Read the model definition and answer for the solid it produces. Units are mm, in the model's axes. A direction names the side the tool comes from. Coordinates: 2 decimals unless noted, no trailing zeros. Order: outer loops, then holes, each group sorted by start corner. A loop starts at its lowest first (then second) coordinate and runs counter-clockwise, first axis right, second up. Notation, with made-up numbers: M -39,-39.75 L -4,-39.75 A8 cw -4,-28.75 Z; hole C 63.25,75 d9. An arc over 180 degrees is marked long. Use a Markdown table: item, result. Add a question column.
1) Find the intervals of material crossed by probe 1 along X at (y, z) = (2, -15); probe 2 along X at (y, z) = (-17, 2.5); probe 3 along X at (y, z) = (1, -6), in increasing order. Write a range as [from, to].
2) Each of these flat-tipped pins is pushed along its axis until it touches: pin 1 Ø2 at (x, z) = (14, -32) entering from -Y; pin 2 Ø9 at (x, z) = (0, -6) entering from +Y; pin 3 Ø4.5 at (x, z) = (-19, -22.5) entering from -Y; pin 4 Ø3 at (y, z) = (-1, -11) entering from -X. Where does it stop, or does it pass through?
3) For faces 5 (the face through (0, 0, -19)), 6 (the face through (24, 11, -35)), 7 (the face through (31.5, 26, 7)), determine the directions among +Z, -Z, +X, -X, +Y, -Y from which every point of the face is accessible in a straight line to the end or side of a thin tool.
4) The mould has two halves that part along Z. Classify faces 1 (the face through (-0.05, -27.25, 3.97)), 2 (the face through (-1.05, 1.6, -3.46)), 3 (the face through (-8, -13, 6)), 4 (the face through (26, 26, 5.5)): released by +Z, released by -Z, zero draft, split by the parting line, or undercut.
5) Find section A-A on y = -22. Write down the section's boundary in (x, z), plus the area to 3 significant figures.
6) Find section D-D on y = 33. Write down the section's boundary in (x, z).
7) Find section C-C on z = -22.5. Write down the section's boundary in (x, y).
8) Find section B-B on x = -19. Write down the section's boundary in (y, z), plus the area to 3 significant figures.
from build123d import *

# Parameters (mm, degrees)
SKETCH1_R           = 2.75
SKETCH1_R_2         = 2.25
BOSS_EXTRUDE1_DEPTH = 4
SKETCH3_W           = 10
SKETCH3_H           = 10
BOSS_EXTRUDE3_DEPTH = 15
SKETCH4_R           = 2.5
CUT_EXTRUDE1_DEPTH  = 58.280013966
CHAMFER1_SIZE       = 0.75
SKETCH5_W           = 4
SKETCH5_H           = 34
BOSS_EXTRUDE4_DEPTH = 68
SKETCH7_R           = 2.75
CUT_EXTRUDE2_DEPTH  = 62.806148561
CHAMFER2_SIZE       = 0.5
SKETCH8_W           = 15
SKETCH8_H           = 10
BOSS_EXTRUDE5_DEPTH = 110
CUT_EXTRUDE3_DEPTH  = 99.346326825
SKETCH10_W          = 10
SKETCH10_H          = 3
CUT_EXTRUDE4_DEPTH  = 122.885191882


with BuildPart() as part:
    # Sketch1 → Boss-Extrude1 (new body)
    with BuildSketch(Plane(origin=(0, 0, 0), x_dir=(1, 0, 0), z_dir=(0, 1, 0))):
        Polygon((-34, 0), (-34, 40), (34, 40), (34, 0), (34, -2), (-34, -2), align=None)
        with Locations(Location((-19, 22.5, 0), (0, 0, 270))):
            Circle(SKETCH1_R, mode=Mode.SUBTRACT)
        with Locations(Location((19, 22.5, 0), (0, 0, 270))):
            Circle(SKETCH1_R, mode=Mode.SUBTRACT)
        with Locations(Location((-29, 15, 0), (0, 0, 270))):
            Circle(SKETCH1_R_2, mode=Mode.SUBTRACT)
        with Locations(Location((29, 15, 0), (0, 0, 270))):
            Circle(SKETCH1_R_2, mode=Mode.SUBTRACT)
        with Locations(Location((0, 6, 0), (0, 0, 270))):
            Circle(SKETCH1_R, mode=Mode.SUBTRACT)
    extrude(amount=BOSS_EXTRUDE1_DEPTH)

    # Sketch3 → Boss-Extrude3 (add)
    with BuildSketch(Plane(origin=(0, 4, 0), x_dir=(1, 0, 0), z_dir=(0, 1, 0))):
        with Locations((-29, 35)):
            Rectangle(SKETCH3_W, SKETCH3_H)
        with Locations((29, 35)):
            Rectangle(SKETCH3_W, SKETCH3_H)
    extrude(amount=BOSS_EXTRUDE3_DEPTH)

    # Sketch4 → Cut-Extrude1 (cut, through all)
    with BuildSketch(Plane(origin=(0, 0, -40), x_dir=(-1, 0, 0), z_dir=(0, 0, -1))):
        with Locations((-29, 12)):
            Circle(SKETCH4_R)
        with Locations((29, 12)):
            Circle(SKETCH4_R)
    extrude(amount=-CUT_EXTRUDE1_DEPTH, mode=Mode.SUBTRACT)

    # Chamfer1
    chamfer1_edges = [part.edges().sort_by_distance(p)[0] for p in [
        (-19, 4, -25.25),
        (19, 4, -25.25),
        (0, 4, -8.75),
    ]]
    chamfer(chamfer1_edges, length=CHAMFER1_SIZE)

    # Sketch5 → Boss-Extrude4 (add)
    with BuildSketch(Plane.ZY.offset(34)):
        with Locations((4, -13)):
            Rectangle(SKETCH5_W, SKETCH5_H)
    extrude(amount=-BOSS_EXTRUDE4_DEPTH)

    # Sketch7 → Cut-Extrude2 (cut, through all)
    with BuildSketch(Plane(origin=(0, 0, 2), x_dir=(-1, 0, 0), z_dir=(0, 0, -1))):
        with Locations(Location((0, -6, 0), (0, 0, 90))):
            Circle(SKETCH7_R)
        with BuildLine():
            Line((2.25, -15), (2.25, -25))
            ThreePointArc((2.25, -25), (0, -27.25), (-2.25, -25))
            Line((-2.25, -25), (-2.25, -15))
            ThreePointArc((-2.25, -15), (0, -12.75), (2.25, -15))
        make_face()
    extrude(amount=-CUT_EXTRUDE2_DEPTH, mode=Mode.SUBTRACT)

    # Chamfer2
    chamfer2_edges = [part.edges().sort_by_distance(p)[0] for p in [
        (0, -8.75, 6),
    ]]
    chamfer(chamfer2_edges, length=CHAMFER2_SIZE)

    # Sketch8 → Boss-Extrude5 (add)
    with BuildSketch(Plane.XZ.offset(30)):
        with Locations((26.5, 7)):
            Rectangle(SKETCH8_W, SKETCH8_H)
    extrude(amount=-BOSS_EXTRUDE5_DEPTH)

    # Sketch9 → Cut-Extrude3 (cut, through all)
    with BuildSketch(Plane.XY.offset(6)):
        with BuildLine():
            Line((19, -3), (19, -24))
            ThreePointArc((19, -24), (17, -26), (15, -24))
            Line((15, -24), (15, -3))
            ThreePointArc((15, -3), (17, -1), (19, -3))
        make_face()
    extrude(amount=-CUT_EXTRUDE3_DEPTH, mode=Mode.SUBTRACT)

    # Sketch10 → Cut-Extrude4 (cut, through all)
    with BuildSketch(Plane(origin=(0, 80, 0), x_dir=(1, 0, 0), z_dir=(0, 1, 0))):
        with Locations((26.5, -7)):
            Rectangle(SKETCH10_W, SKETCH10_H)
    extrude(amount=-CUT_EXTRUDE4_DEPTH, mode=Mode.SUBTRACT)


solid = part.part
Check result:
| question | item | result |
|---|---|---|
| 1 | probe 1 | x = [-34, -31.25], [-26.75, 26.75], [31.25, 34] |
| 1 | probe 2 | x = [-34, -2.25], [2.25, 15], [19, 34] |
| 1 | probe 3 | x = [-34, -2.75], [2.75, 34] |
| 2 | pin 1 | stops at y = 0 |
| 2 | pin 2 | stops at y = 4 |
| 2 | pin 3 | passes through |
| 2 | pin 4 | stops at x = -34 |
| 3 | face 5 | -Z, +X, -X, -Y |
| 3 | face 6 | -Z, +Y |
| 3 | face 7 | +Y, -Y |
| 4 | face 1 | zero draft |
| 4 | face 2 | undercut |
| 4 | face 3 | released by +Z |
| 4 | face 4 | undercut |
| 5 | outline | M -34,2 L -2.25,2 L -2.25,6 L -34,6 Z; M 2.25,2 L 15,2 L 15,6 L 2.25,6 Z; M 19,2 L 34,2 L 34,12 L 19,12 Z; hole M 21.5,5.5 L 31.5,5.5 L 31.5,8.5 L 21.5,8.5 Z |
| 5 | area | 298 mm2 |
| 6 | outline | M 19,2 L 34,2 L 34,12 L 19,12 Z; hole M 21.5,5.5 L 31.5,5.5 L 31.5,8.5 L 21.5,8.5 Z |
| 7 | outline | M -34,0 L -21.75,0 L -21.75,3.25 L -22.5,4 L -34,4 Z; M -16.25,0 L 16.25,0 L 16.25,3.25 L 15.5,4 L -15.5,4 L -16.25,3.25 Z; M 21.75,0 L 34,0 L 34,4 L 22.5,4 L 21.75,3.25 Z |
| 8 | outline | M -30,2 L 0,2 L 0,-19.75 L 3.25,-19.75 L 4,-19 L 4,6 L -30,6 Z; M 0,-40 L 4,-40 L 4,-26 L 3.25,-25.25 L 0,-25.25 Z |
| 8 | area | 281 mm2 |
